from build123d import *

# Parameters (mm, degrees)
BOSS_EXTRUDE1_DEPTH = 2
BOSS_EXTRUDE2_DEPTH = 10
SKETCH3_W           = 7
SKETCH3_H           = 7
SKETCH3_R           = 1.5
BOSS_EXTRUDE3_DEPTH = 4
FILLET1_R           = 5
FILLET2_R           = 3


with BuildPart() as part:
    # Sketch1 → Boss-Extrude1 (new body)
    with BuildSketch(Plane(origin=(0, 0, 0), x_dir=(1, 0, 0), z_dir=(0, 1, 0))):
        with BuildLine():
            Line((-2, 21.835), (-2, -2))
            Line((-2, -2), (89.22, -2))
            Line((89.22, -2), (89.22, 21.835))
            Line((89.22, 21.835), (80.92, 21.835))
            ThreePointArc((80.92, 21.835), (79.22, 20.135), (77.52, 21.835))
            Line((77.52, 21.835), (70.92, 21.835))
            ThreePointArc((70.92, 21.835), (69.22, 20.135), (67.52, 21.835))
            Line((67.52, 21.835), (60.92, 21.835))
            ThreePointArc((60.92, 21.835), (59.22, 20.135), (57.52, 21.835))
            Line((57.52, 21.835), (50.92, 21.835))
            ThreePointArc((50.92, 21.835), (49.22, 20.135), (47.52, 21.835))
            Line((47.52, 21.835), (40.92, 21.835))
            ThreePointArc((40.92, 21.835), (39.22, 20.135), (37.52, 21.835))
            Line((37.52, 21.835), (30.92, 21.835))
            ThreePointArc((30.92, 21.835), (29.22, 20.135), (27.52, 21.835))
            Line((27.52, 21.835), (20.92, 21.835))
            ThreePointArc((20.92, 21.835), (19.22, 20.135), (17.52, 21.835))
            Line((17.52, 21.835), (10.92, 21.835))
            ThreePointArc((10.92, 21.835), (9.22, 20.135), (7.52, 21.835))
            Line((7.52, 21.835), (-2, 21.835))
        make_face()
        with BuildLine():
            Line((-2, 45.67), (-2, 21.835))
            Line((-2, 21.835), (7.52, 21.835))
            ThreePointArc((7.52, 21.835), (9.22, 23.535), (10.92, 21.835))
            Line((10.92, 21.835), (17.52, 21.835))
            ThreePointArc((17.52, 21.835), (19.22, 23.535), (20.92, 21.835))
            Line((20.92, 21.835), (27.52, 21.835))
            ThreePointArc((27.52, 21.835), (29.22, 23.535), (30.92, 21.835))
            Line((30.92, 21.835), (37.52, 21.835))
            ThreePointArc((37.52, 21.835), (39.22, 23.535), (40.92, 21.835))
            Line((40.92, 21.835), (47.52, 21.835))
            ThreePointArc((47.52, 21.835), (49.22, 23.535), (50.92, 21.835))
            Line((50.92, 21.835), (57.52, 21.835))
            ThreePointArc((57.52, 21.835), (59.22, 23.535), (60.92, 21.835))
            Line((60.92, 21.835), (67.52, 21.835))
            ThreePointArc((67.52, 21.835), (69.22, 23.535), (70.92, 21.835))
            Line((70.92, 21.835), (77.52, 21.835))
            ThreePointArc((77.52, 21.835), (79.22, 23.535), (80.92, 21.835))
            Line((80.92, 21.835), (89.22, 21.835))
            Line((89.22, 21.835), (89.22, 45.67))
            Line((89.22, 45.67), (-2, 45.67))
        make_face()
    extrude(amount=BOSS_EXTRUDE1_DEPTH)

    # Sketch2 → Boss-Extrude2 (add)
    with BuildSketch(Plane(origin=(0, 2, 0), x_dir=(1, 0, 0), z_dir=(0, 1, 0))):
        Polygon((-2, 0), (-2, -2), (89.22, -2), (89.22, 45.67), (-2, 45.67), (-2, 43.67), (0, 43.67), (87.22, 43.67), (87.22, 0), (0, 0), align=None)
    extrude(amount=BOSS_EXTRUDE2_DEPTH)

    # Sketch3 → Boss-Extrude3 (add)
    # profile 1 of 4: a face of its own
    with BuildSketch(Plane(origin=(0, 2, 0), x_dir=(1, 0, 0), z_dir=(0, 1, 0))):
        with Locations((81.51878701, 39.735)):
            Rectangle(SKETCH3_W, SKETCH3_H)
        with Locations(Location((81.51878701, 39.735, 0), (0, 0, 270))):
            Circle(SKETCH3_R, mode=Mode.SUBTRACT)
    # profile 2 of 4: a face of its own
    with BuildSketch(Plane(origin=(0, 2, 0), x_dir=(1, 0, 0), z_dir=(0, 1, 0))):
        with Locations((81.51878701, 3.935)):
            Rectangle(SKETCH3_W, SKETCH3_H)
        with Locations(Location((81.51878701, 3.935, 0), (0, 0, 90))):
            Circle(SKETCH3_R, mode=Mode.SUBTRACT)
    # profile 3 of 4: a face of its own
    with BuildSketch(Plane(origin=(0, 2, 0), x_dir=(1, 0, 0), z_dir=(0, 1, 0))):
        with Locations((3.52, 39.3)):
            Rectangle(SKETCH3_W, SKETCH3_H)
        with Locations((3.52, 39.3)):
            Circle(SKETCH3_R, mode=Mode.SUBTRACT)
    # profile 4 of 4: a face of its own
    with BuildSketch(Plane(origin=(0, 2, 0), x_dir=(1, 0, 0), z_dir=(0, 1, 0))):
        with Locations((3.51878701, 3.935)):
            Rectangle(SKETCH3_W, SKETCH3_H)
        with Locations(Location((3.51878701, 3.935, 0), (0, 0, 180))):
            Circle(SKETCH3_R, mode=Mode.SUBTRACT)
    extrude(amount=BOSS_EXTRUDE3_DEPTH)

    # Fillet1
    fillet1_edges = [part.edges().sort_by_distance(p)[0] for p in [
        (-2, 12, -44.67),
        (-2, 12, 1),
    ]]
    fillet(fillet1_edges, radius=FILLET1_R)

    # Fillet2
    fillet2_edges = [part.edges().sort_by_distance(p)[0] for p in [
        (89.22, 6, -45.67),
        (89.22, 6, 2),
    ]]
    fillet(fillet2_edges, radius=FILLET2_R)


solid = part.part
The listing builds one solid part. Answer for the finished solid, in the listing's coordinates (mm). A direction names the side the tool comes from. Coordinates: 2 decimals unless noted, no trailing zeros. Loops run counter-clockwise (first coordinate to the right, second up) from the corner with the lowest first, then second, coordinate; pieces in that order, holes last.
1) Find section B-B on z = -16. Write down the section's boundary in (x, y).
2) Determine the mould class of faces 4 (the face through (41, 6, 2)), 5 (the face through (-1, 10, 1)), 6 (the face through (88.32, 6.08, -44.81)), 7 (the face through (37.6, 0.99, -22.35)) for opening direction Z: pulls with the +Z half, pulls with the -Z half, needs draft (parallel to the pull), parting line crosses it, or undercut.
3) A tool of negligible diameter and unlimited length cuts with its end or side. For faces 1 (the face through (43, 7, 0)), 2 (the face through (3, 2, -39)), 3 (the face through (47.6, 0.99, -22.35)), from which of +Z, -Z, +X, -X, +Y, -Y can it reach the whole face along a straight path? Write none if from no direction.
4) Find section C-C on y = 1. Give the number of separate pieces and of enclosed holes in the cut face, then the cut area to 3 significant figures.
5) Find the intervals of material crossed by L1, parallel to Z at x = 66.5, y = 5.25; L2, parallel to Z at x = 69.22, y = 1.2 (3 decimals); L3, parallel to X at y = 4.5, z = -5, in increasing order.
6) Find section D-D on y = 9. Write down the section's boundary in (x, z).
7) Flat-ended cylindrical pins translate along their axes: pin 1 Ø4 at (x, z) = (70.5, -23.5) entering from +Y; pin 2 Ø3.5 at (x, z) = (81.5, -4.5) entering from +Y; pin 3 Ø5 at (y, z) = (6.5, -22) entering from -X. Find the tip coordinate at first contact, or state that the pin passes through.
8) Find section A-A on x = 69.22. Write down the section's boundary in (y, z) (3 decimals), then the cut area to 3 significant figures.
Values:
1. outline: (-2, 0) - (89.22, 0) - (89.22, 12) - (87.22, 12) - (87.22, 2) - (-2, 2) - close
2. face 4: pulls with the +Z half
2. face 5: needs draft
2. face 6: pulls with the -Z half
2. face 7: undercut
3. face 1: -X, +Y
3. face 2: +Y
3. face 3: +Y, -Y
4. separate pieces: 1
4. enclosed holes: 8
4. area: 4,270 mm2
5. L1: z = -45.67 to -43.67, 0 to 2
5. L2: z = -45.67 to -23.535, -20.135 to 2
5. L3: x = 0.02 to 2.46, 4.58 to 7.02, 78.02 to 80.46, 82.58 to 85.02, 87.22 to 89.22
6. outline: (-1.58, -45.67) - (86.22, -45.67) arc R3 ccw to (89.22, -42.67) - (89.22, -1) arc R3 ccw to (86.22, 2) - (-1.58, 2) - (-1.58, 0) - (87.22, 0) - (87.22, -43.67) - (-1.58, -43.67) - close
7. pin 1: stops at y = 2
7. pin 2: stops at y = 6
7. pin 3: stops at x = 87.22
8. outline: (0, -45.67) - (12, -45.67) - (12, -43.67) - (2, -43.67) - (2, -23.535) - (0, -23.535) - close; (0, -20.135) - (2, -20.135) - (2, 0) - (12, 0) - (12, 2) - (0, 2) - close
8. area: 129 mm2
